The model under review builds one solid part; all positions refer to its coordinate system, in mm. A direction names the side the tool comes from. Round coordinates to 2 decimals unless told otherwise and drop trailing zeros. Order: outer loops, then holes, each group sorted by start corner. A loop starts at its lowest first (then second) coordinate and runs counter-clockwise, first axis right, second up. Notation, with made-up numbers: (41.25, 86) -> (52.25, 86) arc R28 cw to (52.25, 121) -> close; hole circle Ø2 at (2.25, 49). An arc over 180 degrees is marked (long way). Put each result on its own line as item: value. Start each with the question number.
from build123d import *

# Parameters (mm, degrees)
CROQUIS1_W              = 23.5
CROQUIS1_H              = 21.5
SALIENTE_EXTRUIR1_DEPTH = 2.5
CROQUIS2_W              = 15.25
CROQUIS2_H              = 2.5
SALIENTE_EXTRUIR2_DEPTH = 2
CROQUIS4_W              = 11
CROQUIS4_H              = 2
SALIENTE_EXTRUIR4_DEPTH = 1
CROQUIS5_W              = 10
CROQUIS5_H              = 0.5
CORTAR_EXTRUIR1_DEPTH   = 0.75


with BuildPart() as part:
    # Croquis1 → Saliente-Extruir1 (new body)
    with BuildSketch(Plane(origin=(0, 0, 0), x_dir=(1, 0, 0), z_dir=(0, 1, 0))):
        Rectangle(CROQUIS1_W, CROQUIS1_H)
    extrude(amount=SALIENTE_EXTRUIR1_DEPTH)

    # Croquis2 → Saliente-Extruir2 (add)
    with BuildSketch(Plane(origin=(0, 0, -10.75), x_dir=(-1, 0, 0), z_dir=(0, 0, -1))):
        with Locations((0, 1.25)):
            Rectangle(CROQUIS2_W, CROQUIS2_H)
    extrude(amount=SALIENTE_EXTRUIR2_DEPTH)

    # Croquis4 → Saliente-Extruir4 (add)
    with BuildSketch(Plane(origin=(0, 2.5, 0), x_dir=(1, 0, 0), z_dir=(0, 1, 0))):
        with Locations((0, 8.75)):
            Rectangle(CROQUIS4_W, CROQUIS4_H)
    extrude(amount=SALIENTE_EXTRUIR4_DEPTH)

    # Croquis5 → Cortar-Extruir1 (cut)
    with BuildSketch(Plane(origin=(0, 2.5, 0), x_dir=(1, 0, 0), z_dir=(0, 1, 0))):
        with Locations((0, 11.75)):
            Rectangle(CROQUIS5_W, CROQUIS5_H)
    extrude(amount=-CORTAR_EXTRUIR1_DEPTH, mode=Mode.SUBTRACT)


solid = part.part
Q1. Take a section at C-C on z = 5. Give the boundary of the cut face in (x, y), and give its area (4 significant figures).
Q2. Take a section at D-D on y = 2.9. Give the boundary of the cut face in (x, z), and give its area (3 significant figures).
Q3. For faces 1 (the face through (10, 1, -10.75)), 2 (the face through (0, 3, -9.75)), 3 (the face through (-7.625, 1, -12)), list the 3-axis set-ups (+Z, -Z, +X, -X, +Y, -Y) from which the entire face can be reached by the end or side of a thin tool; tool diameter is ignored.
Q4. Wall thickness on probe 1 along Y at (x, z) = (-1, -2.25); probe 2 along Z at (x, y) = (9, 1.5); probe 3 along Z at (x, y) = (1, 3.3): over which ranges is each line inside the solid? List them lowest first. Write a range as [from, to].
Q5. Clearance check with flat-ended pins moving along their axes: pin 1 Ø0.5 at (y, z) = (3, -9) entering from -X; pin 2 Ø1 at (x, z) = (2, -4) entering from +Y; pin 3 Ø0.5 at (x, y) = (0.5, 3) entering from +Z. State where each tip first meets the part, or that it passes through.
Q6. Take a section at B-B on y = 0.5. Give the boundary of the cut face in (x, z) (3 decimals).
Q7. Take a section at A-A on x = -2.5. Give the boundary of the cut face in (y, z), and give its area (3 significant figures).
Calculated:
1. outline: (-11.75, 0) -> (11.75, 0) -> (11.75, 2.5) -> (-11.75, 2.5) -> close
1. area: 58.75 mm²
2. outline: (-5.5, -9.75) -> (5.5, -9.75) -> (5.5, -7.75) -> (-5.5, -7.75) -> close
2. area: 22.0 mm²
3. face 1: -Z, +X, +Y, -Y
3. face 2: -Z, +X, -X, +Y
3. face 3: -Z, -X, +Y, -Y
4. probe 1: y = [0, 2.5]
4. probe 2: z = [-10.75, 10.75]
4. probe 3: z = [-9.75, -7.75]
5. pin 1: stops at x = -5.5
5. pin 2: stops at y = 2.5
5. pin 3: stops at z = -7.75
6. outline: (-11.75, -10.75) -> (-7.625, -10.75) -> (-7.625, -12.75) -> (7.625, -12.75) -> (7.625, -10.75) -> (11.75, -10.75) -> (11.75, 10.75) -> (-11.75, 10.75) -> close
7. outline: (0, -12.75) -> (2.5, -12.75) -> (2.5, -12) -> (1.75, -12) -> (1.75, -11.5) -> (2.5, -11.5) -> (2.5, -9.75) -> (3.5, -9.75) -> (3.5, -7.75) -> (2.5, -7.75) -> (2.5, 10.75) -> (0, 10.75) -> close
7. area: 60.4 mm²
